from build123d import *

# Parameters (mm, degrees)
SKETCH1_R               = 45
SKETCH1_R_2             = 1.5
BOSS_EXTRUDE2_DEPTH     = 5
SKETCH2_R               = 3.96875
BOSS_EXTRUDE3_DEPTH     = 5
SKETCH3_R               = 1.5
CUT_EXTRUDE1_DEPTH      = 7
CUT_EXTRUDE2_DEPTH      = 27
CUT_EXTRUDE2_DEPTH_BACK = 19
SKETCH4_W               = 27.9375
SKETCH4_H               = 5
SKETCH5_W               = 38.057412374
SKETCH5_H               = 36.402742271
BOSS_EXTRUDE4_DEPTH     = 4
SKETCH6_R               = 3.96875
SKETCH6_R_2             = 1.5
BOSS_EXTRUDE5_DEPTH     = 5
CUT_EXTRUDE3_START      = -2
SKETCH6_2_R             = 1.5
CUT_EXTRUDE3_DEPTH      = 2


with BuildPart() as part:
    # Sketch1 → Boss-Extrude2 (new body)
    with BuildSketch(Plane(origin=(0, 0, 0), x_dir=(1, 0, 0), z_dir=(0, 1, 0))):
        with Locations(Location((0, 0, 0), (0, 0, 270))):
            Circle(SKETCH1_R)
        with Locations(Location((0, 41.75, 0), (0, 0, 270))):
            Circle(SKETCH1_R_2, mode=Mode.SUBTRACT)
        with Locations(Location((29.521708115, 29.521708115, 0), (0, 0, 270))):
            Circle(SKETCH1_R_2, mode=Mode.SUBTRACT)
        with Locations(Location((41.75, 0, 0), (0, 0, 270))):
            Circle(SKETCH1_R_2, mode=Mode.SUBTRACT)
        with Locations(Location((29.521708115, -29.521708115, 0), (0, 0, 270))):
            Circle(SKETCH1_R_2, mode=Mode.SUBTRACT)
        with Locations(Location((0, -41.75, 0), (0, 0, 270))):
            Circle(SKETCH1_R_2, mode=Mode.SUBTRACT)
        with Locations(Location((-29.521708115, -29.521708115, 0), (0, 0, 270))):
            Circle(SKETCH1_R_2, mode=Mode.SUBTRACT)
        with Locations(Location((-41.75, 0, 0), (0, 0, 270))):
            Circle(SKETCH1_R_2, mode=Mode.SUBTRACT)
        with Locations(Location((-29.521708115, 29.521708115, 0), (0, 0, 270))):
            Circle(SKETCH1_R_2, mode=Mode.SUBTRACT)
    extrude(amount=BOSS_EXTRUDE2_DEPTH)

    # Sketch2 → Boss-Extrude3 (add)
    with BuildSketch(Plane(origin=(0, 5, 0), x_dir=(1, 0, 0), z_dir=(0, 1, 0))):
        with Locations(Location((-10, 10, 0), (0, 0, 270))):
            Circle(SKETCH2_R)
        with Locations(Location((10, 10, 0), (0, 0, 270))):
            Circle(SKETCH2_R)
        with Locations(Location((10, -10, 0), (0, 0, 270))):
            Circle(SKETCH2_R)
        with Locations(Location((-10, -10, 0), (0, 0, 270))):
            Circle(SKETCH2_R)
    extrude(amount=BOSS_EXTRUDE3_DEPTH)

    # Sketch3 → Cut-Extrude1 (cut)
    with BuildSketch(Plane(origin=(0, 10, 0), x_dir=(1, 0, 0), z_dir=(0, 1, 0))):
        with Locations(Location((-10, 10, 0), (0, 0, 270))):
            Circle(SKETCH3_R)
        with Locations(Location((10, 10, 0), (0, 0, 270))):
            Circle(SKETCH3_R)
        with Locations(Location((-10, -10, 0), (0, 0, 270))):
            Circle(SKETCH3_R)
        with Locations(Location((10, -10, 0), (0, 0, 270))):
            Circle(SKETCH3_R)
    extrude(amount=-CUT_EXTRUDE1_DEPTH, mode=Mode.SUBTRACT)

    # Sketch4 → Cut-Extrude2 (cut, two sides: drawn at the far end of the back side and taken through both)
    with BuildSketch(Plane.XY.offset(-CUT_EXTRUDE2_DEPTH_BACK)):
        with Locations((0, 7.5)):
            Rectangle(SKETCH4_W, SKETCH4_H)
    extrude(amount=CUT_EXTRUDE2_DEPTH + CUT_EXTRUDE2_DEPTH_BACK, mode=Mode.SUBTRACT)

    # Sketch5 → Boss-Extrude4 (add)
    with BuildSketch(Plane(origin=(0, 5, 0), x_dir=(1, 0, 0), z_dir=(0, 1, 0))):
        with Locations((0.472762887, -0.413667525)):
            Rectangle(SKETCH5_W, SKETCH5_H)
    extrude(amount=-BOSS_EXTRUDE4_DEPTH)

    # Sketch6 → Boss-Extrude5 (add)
    # profile 1 of 4: a face of its own
    with BuildSketch(Plane(origin=(0, 5, 0), x_dir=(1, 0, 0), z_dir=(0, 1, 0))):
        with Locations(Location((-15, 15, 0), (0, 0, 270))):
            Circle(SKETCH6_R)
        with Locations(Location((-15, 15, 0), (0, 0, 270))):
            Circle(SKETCH6_R_2, mode=Mode.SUBTRACT)
    # profile 2 of 4: a face of its own
    with BuildSketch(Plane(origin=(0, 5, 0), x_dir=(1, 0, 0), z_dir=(0, 1, 0))):
        with Locations(Location((15, 15, 0), (0, 0, 270))):
            Circle(SKETCH6_R)
        with Locations(Location((15, 15, 0), (0, 0, 270))):
            Circle(SKETCH6_R_2, mode=Mode.SUBTRACT)
    # profile 3 of 4: a face of its own
    with BuildSketch(Plane(origin=(0, 5, 0), x_dir=(1, 0, 0), z_dir=(0, 1, 0))):
        with Locations(Location((15, -15, 0), (0, 0, 270))):
            Circle(SKETCH6_R)
        with Locations(Location((15, -15, 0), (0, 0, 270))):
            Circle(SKETCH6_R_2, mode=Mode.SUBTRACT)
    # profile 4 of 4: a face of its own
    with BuildSketch(Plane(origin=(0, 5, 0), x_dir=(1, 0, 0), z_dir=(0, 1, 0))):
        with Locations(Location((-15, -15, 0), (0, 0, 270))):
            Circle(SKETCH6_R)
        with Locations(Location((-15, -15, 0), (0, 0, 270))):
            Circle(SKETCH6_R_2, mode=Mode.SUBTRACT)
    extrude(amount=BOSS_EXTRUDE5_DEPTH)

    # Sketch6_2 → Cut-Extrude3 (cut)
    with BuildSketch(Plane(origin=(0, 5, 0), x_dir=(1, 0, 0), z_dir=(0, 1, 0)).offset(CUT_EXTRUDE3_START)):
        with Locations(Location((-15, 15, 0), (0, 0, 270))):
            Circle(SKETCH6_2_R)
        with Locations(Location((15, 15, 0), (0, 0, 270))):
            Circle(SKETCH6_2_R)
        with Locations(Location((15, -15, 0), (0, 0, 270))):
            Circle(SKETCH6_2_R)
        with Locations(Location((-15, -15, 0), (0, 0, 270))):
            Circle(SKETCH6_2_R)
    extrude(amount=CUT_EXTRUDE3_DEPTH, mode=Mode.SUBTRACT)


solid = part.part
Design review of the part built by this model. Coordinates are the model's own, in mm. A direction names the side the tool comes from. Coordinates: 2 decimals unless noted, no trailing zeros. Loops run counter-clockwise (first coordinate to the right, second up) from the corner with the lowest first, then second, coordinate; pieces in that order, holes last. Notation, with made-up numbers: (52.5, -20.5) - (82.5, -20.5) arc R5 cw to (82.5, -12.5) - close; hole circle Ø1 at (83.5, 63). An arc over 180 degrees is marked (long way). Use CSV: the item, a comma, the result in double quotes. Start each with the question number.
1. Add section D-D on z = 41.75. Give the boundary of the cut face in (x, y).
2. Mouldability with a two-part tool opening along X and no side actions: class faces 3 (the cylindrical face through (29.588, 2.465, 28.023)), 4 (the cylindrical face through (-17.235, 2.465, 41.569)), 5 (the flat face through (1, 0, -1)) as released by +X, released by -X, zero draft, split by the parting line, or undercut.
3. To check wall thickness, follow probe 1 along X at (y, z) = (6.5, -15); probe 2 along X at (y, z) = (2.55, 0); probe 3 along X at (y, z) = (2.5, 30). State the ranges of each line that lie inside material, in increasing order.
4. Clearance check with flat-ended pins moving along their axes: pin 1 (6 mm diameter, centred on y = 2.5, z = -15.5, fed in from -X); pin 2 (5 mm diameter, centred on x = 0, z = 41.75, fed in from +Y); pin 3 (3 mm diameter, centred on x = -14, y = 5, fed in from -Z). State where each tip first meets the part, or that it passes through.
5. Add section A-A on y = 6.5. Give the boundary of the cut face in (x, z).
6. Add section B-B on z = 0. Give the boundary of the cut face in (x, y).
7. Add section C-C on x = 41.75. Give the boundary of the cut face in (y, z), plus the area to 3 significant figures.
8. For faces 1 (the cylindrical face through (-11.65, 7.46, -12.87)), 2 (the cylindrical face through (-30.852, 2.465, -28.83)), list the 3-axis set-ups (+Z, -Z, +X, -X, +Y, -Y) from which the entire face can be reached by the end or side of a thin tool; tool diameter is ignored.
Resolved:
1,outline,"(-16.79, 0) - (-1.5, 0) - (-1.5, 5) - (-16.79, 5) - close; (1.5, 0) - (16.79, 0) - (16.79, 5) - (1.5, 5) - close"
2,face 3,"undercut"
2,face 4,"split by the parting line"
2,face 5,"zero draft"
3,probe 1,"-18.97 to -16.5, -13.5 to -11.03, 11.03 to 13.5, 16.5 to 18.97"
3,probe 2,"-45 to -43.25, -40.25 to 40.25, 43.25 to 45"
3,probe 3,"-33.54 to -30.94, -28.1 to 28.1, 30.94 to 33.54"
4,pin 1,"x = -43.23"
4,pin 2,"y = 5"
4,pin 3,"z = -43.23"
5,outline,"circle Ø7.94 at (-15, -15); circle Ø7.94 at (-15, 15); circle Ø7.94 at (15, -15); circle Ø7.94 at (15, 15); hole circle Ø3 at (-15, -15); hole circle Ø3 at (-15, 15); hole circle Ø3 at (15, -15); hole circle Ø3 at (15, 15)"
6,outline,"(-45, 0) - (-43.25, 0) - (-43.25, 5) - (-45, 5) - close; (-40.25, 0) - (40.25, 0) - (40.25, 5) - (-40.25, 5) - close; (43.25, 0) - (45, 0) - (45, 5) - (43.25, 5) - close"
7,outline,"(0, -16.79) - (5, -16.79) - (5, -1.5) - (0, -1.5) - close; (0, 1.5) - (5, 1.5) - (5, 16.79) - (0, 16.79) - close"
7,area,"153 mm2"
8,face 1,"+Y"
8,face 2,"+Y, -Y"
